Check sheet for the modelled part. Datum: model origin and axes. Units: mm. A direction names the side the tool comes from. Give positions to 0.01 mm unless a question says otherwise; leave off trailing zeros. Write each loop counter-clockwise with the first axis right and the second up, starting at its lowest first coordinate (ties: lowest second). Pieces come first, ordered by that corner, then holes. Notation, with made-up numbers: (7, 7.5) -> (40, 7.5) arc R22 cw to (40, 23.5) -> close; hole circle Ø2 at (-27.75, 85.25). An arc over 180 degrees is marked (long way). Write each question's results on one line, items separated by ' | '. Start each with the question number.
```python
from build123d import *

# Parameters (mm, degrees)
EXTRUDE_1_DEPTH     = 43
SKETCH_2_W          = 10
SKETCH_2_H          = 17
CUT_EXTRUDE_1_DEPTH = 43
EXTRUDE_2_DEPTH     = 30
SKETCH_5_W          = 15
SKETCH_5_H          = 4
CUT_EXTRUDE_3_DEPTH = 99.440034066
CUT_EXTRUDE_4_DEPTH = 99.440034066
FILLET_1_R          = 2
FILLET_START        = 0.132447056
FILLET_2_DEPTH      = 43.867552944
FILLET_3_R          = 2
SKETCH_7_W          = 7
SKETCH_7_H          = 15
CUT_EXTRUDE_5_DEPTH = 17
FILLET_4_R          = 2


with BuildPart() as part:
    # Эскиз1 → Бобышка-Вытянуть1 (new body)
    with BuildSketch(Plane.XY):
        Polygon((-61.18540146, 10.360583942), (68.81459854, 10.360583942), (68.81459854, 35.360583942), (78.81459854, 27.459854015), (78.81459854, 0.360583942), (-71.18540146, 0.360583942), (-71.18540146, 27.459854015), (-61.18540146, 35.360583942), align=None)
    extrude(amount=EXTRUDE_1_DEPTH)

    # Эскиз2 → Вырез-Вытянуть1 (cut)
    with BuildSketch(Plane(origin=(-61.18540146, 0, 0), x_dir=(0, 0, -1), z_dir=(1, 0, 0))):
        with Locations((-38, 26.860583942)):
            Rectangle(SKETCH_2_W, SKETCH_2_H)
    extrude(amount=-CUT_EXTRUDE_1_DEPTH, mode=Mode.SUBTRACT)

    # Эскиз3 → Бобышка-Вытянуть2 (add)
    with BuildSketch(Plane.XY):
        Polygon((-71.18540146, 18.360583942), (-71.18540146, 22.873529361), (-81.18540146, 22.873529361), (-81.18540146, 18.360583942), (-81.18540146, 4.73264295), (-71.18540146, 4.73264295), align=None)
    extrude(amount=EXTRUDE_2_DEPTH)

    # Эскиз5 → Вырез-Вытянуть3 (cut, through all)
    with BuildSketch(Plane.XY.offset(43)):
        with Locations((2.81459854, 5.360583942)):
            Rectangle(SKETCH_5_W, SKETCH_5_H)
        with Locations((-44.18540146, 5.360583942)):
            Rectangle(SKETCH_5_W, SKETCH_5_H)
        with Locations((49.81459854, 5.360583942)):
            Rectangle(SKETCH_5_W, SKETCH_5_H)
    extrude(amount=-CUT_EXTRUDE_3_DEPTH, mode=Mode.SUBTRACT)

    # Эскиз6 → Вырез-Вытянуть4 (cut, through all)
    with BuildSketch(Plane.XY.offset(43)):
        Polygon((71.115819654, 30.345691142), (75.823743696, 26.626087505), (75.823743696, 22.626087505), (71.115819654, 26.345691142), align=None)
        Polygon((71.115819654, 19.973455793), (75.823743696, 16.253852156), (75.823743696, 12.253852156), (71.115819654, 15.973455793), align=None)
        Polygon((71.115819654, 9.601220443), (75.823743696, 5.881616806), (75.823743696, 1.881616806), (71.115819654, 5.601220443), align=None)
    extrude(amount=-CUT_EXTRUDE_4_DEPTH, mode=Mode.SUBTRACT)

    # Скругление1
    fillet_1_edges = [part.edges().sort_by_distance(p)[0] for p in [
        (78.81459854, 27.459854015, 21.5),
        (78.81459854, 0.360583942, 21.5),
        (-71.18540146, 27.459854015, 16.5),
    ]]
    fillet(fillet_1_edges, radius=FILLET_1_R)

    # Скругление2: read off the stored shape, not the designer's step
    # Скругление2 outline → Скругление2 (cut)
    with BuildSketch(Plane.XY.offset(FILLET_START)):
        with BuildLine():
            Line((-71.18540146, 0.360583942), (-69.18540146, 0.360583942))
            ThreePointArc((-69.18540146, 0.360583942), (-70.599615022, 0.94637038), (-71.18540146, 2.360583942))
            Line((-71.18540146, 2.360583942), (-71.18540146, 0.360583942))
        make_face()
    extrude(amount=FILLET_2_DEPTH, mode=Mode.SUBTRACT)

    # Скругление3
    fillet_3_edges = [part.edges().sort_by_distance(p)[0] for p in [
        (-66.18540146, 18.360583942, 43),
        (-66.18540146, 18.360583942, 33),
    ]]
    fillet(fillet_3_edges, radius=FILLET_3_R)

    # Эскиз7 → Вырез-Вытянуть5 (cut)
    with BuildSketch(Plane.XY.offset(30)):
        with Locations((-73.719422713, 13.759023225)):
            Rectangle(SKETCH_7_W, SKETCH_7_H)
    extrude(amount=-CUT_EXTRUDE_5_DEPTH, mode=Mode.SUBTRACT)

    # Скругление4
    fillet_4_edges = [part.edges().sort_by_distance(p)[0] for p in [
        (-81.18540146, 4.73264295, 15),
        (-71.18540146, 4.73264295, 15),
        (-71.18540146, 22.873529361, 15),
        (-81.18540146, 22.873529361, 15),
    ]]
    fillet(fillet_4_edges, radius=FILLET_4_R)


solid = part.part
```
Item 1: Section check A-A on x = -40. Record the boundary of the cut face in (y, z).
Item 2: Mould release check, pull along X, two halves, no side actions. Record for faces 6 (the flat face through (78.815, 15, 21)), 7 (the flat face through (-74, 21.259, 22)), 8 (the flat face through (-76, 22.874, 15)): pulls with the +X half, pulls with the -X half, needs draft (parallel to the pull), parting line crosses it, or undercut.
Item 3: Set-up check for faces 1 (the flat face through (73.37, 31.76, 21.2)), 2 (the flat face through (-66, 18.361, 38)), 3 (the flat face through (3, 3.361, 22)), 4 (the flat face through (-61.185, 23, 16)), 5 (the flat face through (-70.219, 14, 22)): record each of +Z, -Z, +X, -X, +Y, -Y from which the full face is reachable in a straight line by a thin tool's end or side.
Item 4: Section check B-B on z = 14.5. Count the separate pieces of the cut face and the enclosed holes in it, then the cut area to 3 significant figures.
Item 5: Depth check by flat-ended pin: pin 1 Ø16.5 at (x, z) = (3, 20) entering from +Y; pin 2 Ø6.5 at (x, z) = (-66.5, 38.5) entering from +Y; pin 3 Ø1.5 at (y, z) = (4.5, 31) entering from -X. Enter the tip coordinate at first touch or a pass-through.
Item 6: Thickness scan on probe 1 along X at (y, z) = (16, 24); probe 2 along Y at (x, z) = (52.5, 40.5); probe 3 along X at (y, z) = (29.5, 25.5). Record the ranges inside material, lowest first. Write a range as from..to.
Item 7: Section check D-D on x = -6.5. Record the boundary of the cut face in (y, z).
Check sheet entries:
1) outline: (0.36, 0) -> (3.36, 0) -> (3.36, 43) -> (0.36, 43) -> close; (7.36, 0) -> (10.36, 0) -> (10.36, 43) -> (7.36, 43) -> close
2) face 6: pulls with the +X half | face 7: undercut | face 8: needs draft
3) face 1: +Z, -Z, +X, +Y | face 2: +Z, -X, +Y | face 3: +Z, -Z | face 4: +Z, -Z, +Y | face 5: none
4) separate pieces: 1 | enclosed holes: 7 | area: 1,760 mm^2
5) pin 1: stops at y = 10.36 | pin 2: stops at y = 18.36 | pin 3: stops at x = -71.19
6) probe 1: x = -81.19..-77.22, -70.22..-61.19, 68.81..71.12, 75.82..78.81 | probe 2: y = 0.36..3.36, 7.36..10.36 | probe 3: x = -68.6..-61.19, 68.81..71.12, 72.19..76.23
7) outline: (0.36, 0) -> (10.36, 0) -> (10.36, 43) -> (0.36, 43) -> close
